Can you work these out from the model? Positions are in its coordinate system, mm. Give positions to 0.01 mm unless a question says otherwise; leave off trailing zeros. Loops run counter-clockwise (first coordinate to the right, second up) from the corner with the lowest first, then second, coordinate; pieces in that order, holes last. Notation, with made-up numbers: (-31.5, 12.5) - (-15.5, 12.5) arc R19 cw to (-15.5, 35.5) - close; hole circle Ø8 at (58, 38). An arc over 180 degrees is marked (long way). Answer as a JSON object with one key per item and string values. Group by question number.
Item 1: Please list where these lines run through material, in increasing order: L1, parallel to Y at x = -13.5, z = 58.5; L2, parallel to Y at x = 28.5, z = 25; L3, parallel to Z at x = -27, y = 14.
Item 2: Suppose I cut it at C-C on z = 29. Write out the boundary of the cut face in (x, y), and give its area (3 significant figures).
Item 3: Suppose I cut it at A-A on x = -29. Write out the boundary of the cut face in (y, z), and give its area (3 significant figures).
Item 4: Suppose I cut it at B-B on y = -28.5. Write out the boundary of the cut face in (x, z), and give its area (3 significant figures).
Item 5: Will these pins go through, and if not, where does the flat tip stop? pin 1 (1.5 mm diameter, centred on x = 23.5, z = 48, fed in from -Y); pin 2 (8 mm diameter, centred on x = 36, y = 23.5, fed in from -Z); pin 3 (3 mm diameter, centred on x = 30.5, y = 9.5, fed in from +Z); pin 4 (12 mm diameter, centred on x = 10, y = 8.5, fed in from +Z).
from build123d import *

# Parameters (mm, degrees)
SKETCH_W          = 91.5
SKETCH_H          = 95.5
PAD_DEPTH         = 60.5
POCKET_DEPTH      = 45.751
POCKET_DEPTH_BACK = 45.751
FILLET_R          = 10


with BuildPart() as part:
    # Sketch (on XY_Plane of Origin) → Pad (new body)
    with BuildSketch(Plane.XY):
        Rectangle(SKETCH_W, SKETCH_H)
    extrude(amount=PAD_DEPTH)

    # Sketch001 (on YZ_Plane of Origin) → Pocket (cut, two sides)
    with BuildSketch(Plane.YZ) as pocket_sk:
        Polygon((-47.75, 22), (41.028192, 60.5), (47.75, 45), (57.75, 45), (57.75, 70.5), (-57.75, 70.5), (-57.75, 22), align=None)
    extrude(amount=-POCKET_DEPTH, mode=Mode.SUBTRACT)
    extrude(pocket_sk.sketch, amount=POCKET_DEPTH_BACK, mode=Mode.SUBTRACT)

    # Fillet
    fillet_edges = [part.edges().sort_by_distance(p)[0] for p in [
        (45.75, -47.75, 11),
        (-45.75, -47.75, 11),
    ]]
    fillet(fillet_edges, radius=FILLET_R)


solid = part.part
Worked out:
{
 "1": {"L1": "y = 36.42 to 41.9", "L2": "y = -40.83 to 47.75", "L3": "z = 0 to 48.78"},
 "2": {"outline": "(-45.75, -31.61) - (45.75, -31.61) - (45.75, 47.75) - (-45.75, 47.75) - close", "area": "7,260 mm2"},
 "3": {"outline": "(-47.75, 0) - (47.75, 0) - (47.75, 45) - (41.03, 60.5) - (-47.75, 22) - close", "area": "4,020 mm2"},
 "4": {"outline": "(-45.75, 0) - (45.75, 0) - (45.75, 30.35) - (-45.75, 30.35) - close", "area": "2,780 mm2"},
 "5": {"pin 1": "stops at y = 10.47", "pin 2": "stops at z = 0", "pin 3": "stops at z = 47.48", "pin 4": "stops at z = 49"}
}
